Input: part model. Units: mm. Frame: model coordinates. Face numbers are marked on the shaded views. A direction names the side the tool comes from. Coordinates: 2 decimals unless noted, no trailing zeros. Loops run counter-clockwise (first coordinate to the right, second up) from the corner with the lowest first, then second, coordinate; pieces in that order, holes last.
(1) Section C-C, the plane x = 3.75. Return loops of the section in (y, z), then the cut area to 3 significant figures.
(2) Set-up query: the marked faces 4 and 5. Return all of +Z, -Z, +X, -X, +Y, -Y with unobstructed straight access to the full face (end or side cutting, diameter ignored); none if empty.
(3) Section A-A, the plane y = -2. Give the number of separate pieces and of enclosed holes in the cut face, then the cut area to 3 significant figures.
(4) Contact query for flat-ended pins moving along their axis: P1, Ø1.1, axis at x = 0, y = -2, coming from the -Z side; P2, Ø1.8, axis at y = -2.5, z = 0.5, coming from the -X side; P3, Ø4, axis at y = 14, z = -1, coming from the -X side; P4, Ø4, axis at x = -1.5, z = 1, coming from the -Y side. Output: stop coordinate, or through.
(5) Line query: L1, parallel to X at y = 15.4, z = 0; L2, parallel to X at y = 16.3, z = 0. Output: solid intervals per line, ascending.
(6) Section D-D, the plane y = 16.5. Return loops of the section in (x, z).
(7) Mould query, pull axis Y, two halves, no side actions, for the marked faces 1, 2 and 3. Classes: released by +Y, released by -Y, zero draft, split by the parting line, or undercut.
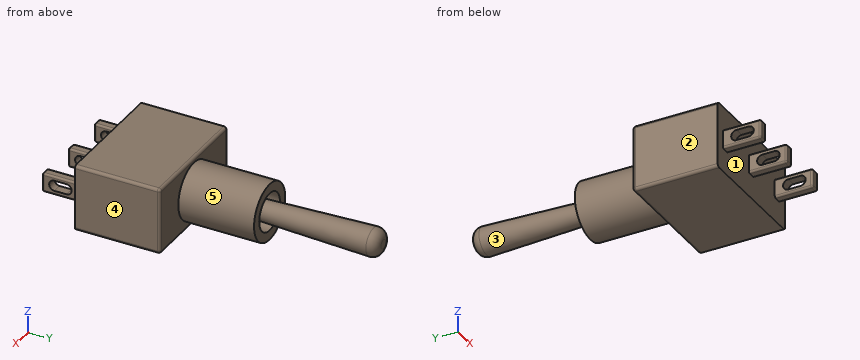
```python
from build123d import *

# Parameters (mm, degrees)
SKETCH1_W           = 13
SKETCH1_H           = 7
SKETCH1_W_2         = 1
SKETCH1_H_2         = 2
BOSS_EXTRUDE1_DEPTH = 9
SKETCH1_3_W         = 1
SKETCH1_3_H         = 2
BOSS_EXTRUDE2_DEPTH = 4
SKETCH2_R           = 3
SKETCH2_R_2         = 2
BOSS_EXTRUDE3_DEPTH = 8
SKETCH2_6_R         = 2
BOSS_EXTRUDE4_DEPTH = 5
SKETCH4_R           = 1
SKETCH3_R           = 1.5
FILLET1_R           = 1
CUT_EXTRUDE1_DEPTH  = 12
FILLET2_R           = 0.3
FILLET3_R           = 0.2


with BuildPart() as part:
    # Sketch1 → Boss-Extrude1 (new body)
    with BuildSketch(Plane(origin=(0, 0, 0), x_dir=(1, 0, 0), z_dir=(0, 1, 0))):
        Rectangle(SKETCH1_W, SKETCH1_H)
        Rectangle(SKETCH1_W_2, SKETCH1_H_2, mode=Mode.SUBTRACT)
        with Locations((-5, 0)):
            Rectangle(SKETCH1_W_2, SKETCH1_H_2, mode=Mode.SUBTRACT)
        with Locations((5, 0)):
            Rectangle(SKETCH1_W_2, SKETCH1_H_2, mode=Mode.SUBTRACT)
        with Locations((-5, 0)):
            Rectangle(SKETCH1_W_2, SKETCH1_H_2)
        Rectangle(SKETCH1_W_2, SKETCH1_H_2)
        with Locations((5, 0)):
            Rectangle(SKETCH1_W_2, SKETCH1_H_2)
    extrude(amount=BOSS_EXTRUDE1_DEPTH)

    # Sketch1_3 → Boss-Extrude2 (add)
    with BuildSketch(Plane(origin=(0, 0, 0), x_dir=(1, 0, 0), z_dir=(0, 1, 0))):
        with Locations((-5, 0)):
            Rectangle(SKETCH1_3_W, SKETCH1_3_H)
        Rectangle(SKETCH1_3_W, SKETCH1_3_H)
        with Locations((5, 0)):
            Rectangle(SKETCH1_3_W, SKETCH1_3_H)
    extrude(amount=-BOSS_EXTRUDE2_DEPTH)

    # Sketch2 → Boss-Extrude3 (add)
    with BuildSketch(Plane(origin=(0, 9, 0), x_dir=(1, 0, 0), z_dir=(0, 1, 0))):
        Circle(SKETCH2_R)
        Circle(SKETCH2_R_2, mode=Mode.SUBTRACT)
    extrude(amount=BOSS_EXTRUDE3_DEPTH)

    # Sketch2_6 → Boss-Extrude4 (add)
    with BuildSketch(Plane(origin=(0, 9, 0), x_dir=(1, 0, 0), z_dir=(0, 1, 0))):
        Circle(SKETCH2_6_R)
    extrude(amount=BOSS_EXTRUDE4_DEPTH)

    # Sketch4 → Loft1 section 0
    with BuildSketch(Plane(origin=(0, 14, 0), x_dir=(1, 0, 0), z_dir=(0, 1, 0))):
        Circle(SKETCH4_R)
    # Sketch3 → Loft1 section 1
    with BuildSketch(Plane(origin=(0, 29, 0), x_dir=(1, 0, 0), z_dir=(0, 1, 0))):
        Circle(SKETCH3_R)
    loft()

    # Fillet1
    fillet1_edges = [part.edges().sort_by_distance(p)[0] for p in [
        (-1.5, 29, 0),
    ]]
    fillet(fillet1_edges, radius=FILLET1_R)

    # Sketch5 → Cut-Extrude1 (cut)
    with BuildSketch(Plane.ZY.offset(5.5)):
        with BuildLine():
            Line((0.550014323, -1.43369619), (0.550014323, -2.717062944))
            ThreePointArc((0.550014323, -2.717062944), (0, -3.267077268), (-0.550014323, -2.717062944))
            Line((-0.550014323, -2.717062944), (-0.550014323, -1.43369619))
            ThreePointArc((-0.550014323, -1.43369619), (0, -0.883681867), (0.550014323, -1.43369619))
        make_face()
    extrude(amount=-CUT_EXTRUDE1_DEPTH, mode=Mode.SUBTRACT)

    # Fillet2
    fillet2_edges = [part.edges().sort_by_distance(p)[0] for p in [
        (0, 9, -3.5),
        (-6.5, 9, 0),
        (0, 9, 3.5),
        (6.5, 9, 0),
        (6.5, 4.5, 3.5),
        (-6.5, 4.5, 3.5),
        (-6.5, 4.5, -3.5),
        (6.5, 4.5, -3.5),
    ]]
    fillet(fillet2_edges, radius=FILLET2_R)

    # Fillet3
    fillet3_edges = [part.edges().sort_by_distance(p)[0] for p in [
        (-4.5, -2, -1),
        (-5, -4, 1),
        (-4.5, -2, 1),
        (-5.5, -4, 0),
        (-5.5, -2, 1),
        (-5.5, -2, -1),
        (-4.5, -4, 0),
        (-5, -4, -1),
        (0.5, -2, -1),
        (0, -4, 1),
        (0.5, -2, 1),
        (-0.5, -4, 0),
        (-0.5, -2, 1),
        (-0.5, -2, -1),
        (0.5, -4, 0),
        (0, -4, -1),
        (5.5, -2, 1),
        (4.5, -4, 0),
        (4.5, -2, 1),
        (5, -4, -1),
        (4.5, -2, -1),
        (5.5, -2, -1),
        (5, -4, 1),
        (5.5, -4, 0),
    ]]
    fillet(fillet3_edges, radius=FILLET3_R)


solid = part.part
```
Report:
1. outline: (0, -3.5) - (8.7, -3.5) arc R0.3 ccw to (9, -3.2) - (9, 3.2) arc R0.3 ccw to (8.7, 3.5) - (0, 3.5) - close
1. area: 63.0 mm2
2. face 4: +Z, -Z, +X, +Y, -Y
2. face 5: +Y
3. separate pieces: 6
3. enclosed holes: 0
3. area: 2.60 mm2
4. P1: stops at z = -1
4. P2: stops at x = -5.5
4. P3: stops at x = -3
4. P4: stops at y = -4
5. L1: x = -3 to -2, -1.05 to 1.05, 2 to 3
5. L2: x = -3 to -2, -1.08 to 1.08, 2 to 3
6. outline: circle Ø6 at (0, 0); circle Ø2.17 at (0, 0); hole circle Ø4 at (0, 0)
7. face 1: released by -Y
7. face 2: zero draft
7. face 3: undercut
